```python
from build123d import *

# Parameters (mm, degrees)
F0_W     = 19.05
F0_H     = 50.8
F0_R     = 4.7625
F1_DEPTH = 6.35
F2_R     = 9.52499


# Not quite as in the source:
# - a fillet or chamfer is up to 0.001 mm smaller than in the source, because OpenCascade refuses the exact size


with BuildPart() as f1:
    # F0 (on Right) → F1 (new body)
    with BuildSketch(Plane.YZ):
        Rectangle(F0_W, F0_H)
        with Locations((0, -19.05)):
            Circle(F0_R, mode=Mode.SUBTRACT)
        with Locations((0, 19.05)):
            Circle(F0_R, mode=Mode.SUBTRACT)
    extrude(amount=F1_DEPTH)

    # F2 (radius 9.525 in the source; OpenCascade refuses exactly that, so slightly less here)
    f2_edges = [f1.edges().sort_by_distance(p)[0] for p in [
        (3.175, 9.525, 25.4),
        (3.175, -9.525, 25.4),
        (3.175, 9.525, -25.4),
        (3.175, -9.525, -25.4),
    ]]
    fillet(f2_edges, radius=F2_R)


solid = f1.part
```
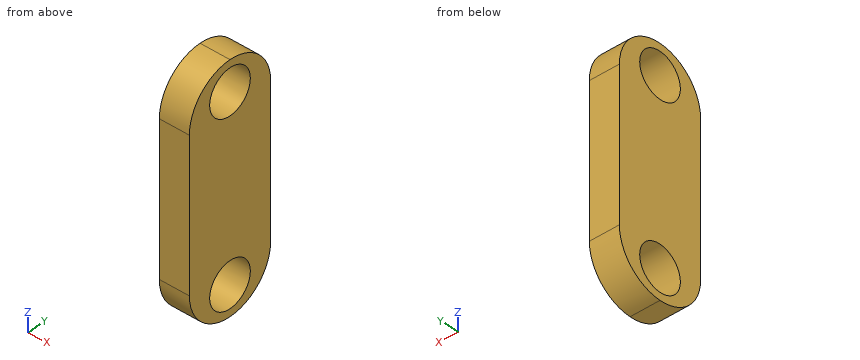
Read the model definition and answer for the solid it produces. Units are mm, in the model's axes. Give positions to 0.01 mm unless a question says otherwise; leave off trailing zeros. Order: outer loops, then holes, each group sorted by start corner. A loop starts at its lowest first (then second) coordinate and runs counter-clockwise, first axis right, second up. Notation, with made-up numbers: (74, 47) -> (112, 47) arc R27 cw to (112, 78) -> close; hole circle Ø11 at (-1.75, 44). An arc over 180 degrees is marked (long way). Write item = value, one per line.
1. A cutting plane is placed at D-D, the plane y = 7.75. Write down the section's boundary in (x, z), and give its area (3 significant figures).
Numbers:
outline = (0, -21.41) -> (6.35, -21.41) -> (6.35, 21.41) -> (0, 21.41) -> close
area = 272 mm²
2. A cutting plane is placed at B-B, the plane z = -19.05. Write down the section's boundary in (x, y).
Numbers:
outline = (0, -8.98) -> (6.35, -8.98) -> (6.35, -4.76) -> (0, -4.76) -> close; (0, 4.76) -> (6.35, 4.76) -> (6.35, 8.98) -> (0, 8.98) -> close
3. A cutting plane is placed at A-A, the plane x = 4.75. Count the separate pieces of the cut face and the enclosed holes in it, and give its area (3 significant figures).
Numbers:
separate_pieces = 1
enclosed_holes = 2
area = 747 mm²
4. Straight lines are drawn through the part: line 1 along Z through (x, y) = (2.25, 0); line 2 along Z through (x, y) = (3.75, -4); line 3 along Y through (x, z) = (1, -23). For each, find the intervals that lie inside material, in ascending order.
Numbers:
line_1 = -25.4 to -23.81, -14.29 to 14.29, 23.81 to 25.4
line_2 = -24.52 to -21.63, -16.47 to 16.47, 21.63 to 24.52
line_3 = -6.32 to -2.66, 2.66 to 6.32
5. A cutting plane is placed at C-C, the plane y = 4. Write down the section's boundary in (x, z).
Numbers:
outline = (0, -24.52) -> (6.35, -24.52) -> (6.35, -21.63) -> (0, -21.63) -> close; (0, -16.47) -> (6.35, -16.47) -> (6.35, 16.47) -> (0, 16.47) -> close; (0, 21.63) -> (6.35, 21.63) -> (6.35, 24.52) -> (0, 24.52) -> close
6. Given pin 1 (3 mm diameter, centred on x = 1.5, y = 6, fed in from +Z); pin 2 (1 mm diameter, centred on x = 3.5, z = 18.5, fed in from +Y); pin 3 (11 mm diameter, centred on y = 0, z = -19.05, fed in from -X), each flat-ended and moving along its own axis, determine where each tip first touches the part or whether it passes through.
Numbers:
pin_1 = 24.27
pin_2 = 9.28
pin_3 = 0
